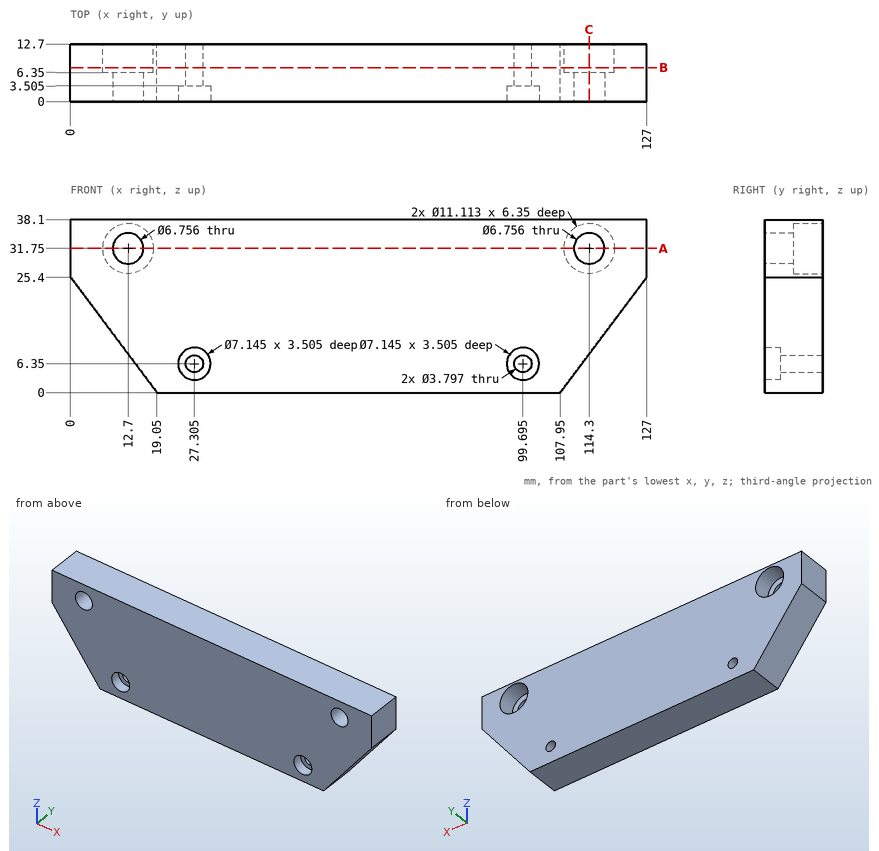
Source: three-view drawing plus pictorial views. Frame: mm from the lowest corner of the part. Round coordinates to 2 decimals unless told otherwise and drop trailing zeros. Loops run counter-clockwise (first coordinate to the right, second up) from the corner with the lowest first, then second, coordinate; pieces in that order, holes last.
1. Section query B-B on y = 7.5. Give the number of separate pieces and of enclosed holes in the cut face, and give its area (3 significant figures).
2. Section query A-A on z = 31.75. Output: boundary loops of the cut face in (x, y).
3. Section query C-C on x = 114.3. Output: boundary loops of the cut face in (y, z), and give its area (3 significant figures).
4. Contact query for flat-ended pins moving along their axis: pin 1 (10 mm diameter, centred on x = 12.7, z = 31.75, fed in from -Y); pin 2 (5 mm diameter, centred on y = 1.5, z = 10, fed in from -X) (1 decimal); pin 3 (9 mm diameter, centred on x = 12.7, z = 31.75, fed in from +Y). Output: stop coordinate, or through.
5. Ray query, L1, parallel to X at y = 5, z = 29 (1 decimal); L2, parallel to X at y = 5.75, z = 6.5 (1 decimal); L3, parallel to Y at x = 113, z = 35.5. Return the intervals inside material, ascending.
Answers below:
1. separate pieces: 1
1. enclosed holes: 4
1. area: 4,140 mm2
2. outline: (0, 0) - (9.32, 0) - (9.32, 6.35) - (7.14, 6.35) - (7.14, 12.7) - (0, 12.7) - close; (16.08, 0) - (110.92, 0) - (110.92, 6.35) - (108.74, 6.35) - (108.74, 12.7) - (18.26, 12.7) - (18.26, 6.35) - (16.08, 6.35) - close; (117.68, 0) - (127, 0) - (127, 12.7) - (119.86, 12.7) - (119.86, 6.35) - (117.68, 6.35) - close
3. outline: (0, 8.47) - (12.7, 8.47) - (12.7, 26.19) - (6.35, 26.19) - (6.35, 28.37) - (0, 28.37) - close; (0, 35.13) - (6.35, 35.13) - (6.35, 37.31) - (12.7, 37.31) - (12.7, 38.1) - (0, 38.1) - close
3. area: 263 mm2
4. pin 1: stops at y = 0
4. pin 2: stops at x = 9.7
4. pin 3: stops at y = 6.35
5. L1: x = 0 to 10.7, 14.7 to 112.3, 116.3 to 127
5. L2: x = 14.2 to 25.4, 29.2 to 97.8, 101.6 to 112.8
5. L3: y = 0 to 6.35
